For this review, take the finished solid that the model builds, in its own axes (mm). Face numbers are marked on the shaded views. A direction names the side the tool comes from. Coordinates: 2 decimals unless noted, no trailing zeros. Order: outer loops, then holes, each group sorted by start corner. A loop starts at its lowest first (then second) coordinate and runs counter-clockwise, first axis right, second up. Notation, with made-up numbers: (15.5, 48) -> (46.5, 48) arc R25 cw to (46.5, 79) -> close; hole circle Ø9 at (67.5, 81.5). An arc over 180 degrees is marked (long way). Return JSON: item names as keys, results as strings. Group by question number.
Item 1: Take a section at C-C (y = -26). Write out the cut boundary in (x, z).
Item 2: For line 1 along Y through (x, z) = (-312, 6); line 2 along X through (y, z) = (-67, 11); line 3 along Z through (x, y) = (312, -68), list the stretches that pass through material, from the lowest coordinate up.
Item 3: Take a section at B-B (x = 178.5). Write out the cut boundary in (y, z), then the cut area to 3 significant figures.
Item 4: Draft analysis for pull direction Z (two halves, no side actions). For the marked faces 1 and 2, state which applies: +Z half, -Z half, draft (parallel to the pull), parting line (faces both ways), or undercut.
Item 5: Take a section at D-D (z = 59.5). Write out the cut boundary in (x, y).
Item 6: Machinability: for the marked faces 3 and 4, which of the approach directions +Z, -Z, +X, -X, +Y, -Y give a long, thin tool a straight path to every point of the face, cutting with its end or side? Answer none if there is none.
Item 7: Take a section at A-A (y = -51). Write out the cut boundary in (x, z).
Item 8: Insertion check: pin 1 (4 mm diameter, centred on x = -326, z = 4, fed in from +Y); pin 2 (4 mm diameter, centred on x = 2, z = 13, fed in from -Y); pin 3 (0.8 mm diameter, centred on x = 312, y = -76.5, fed in from +Z). Each pin has a flat end and moves straight along its axis. Give the tip position at first contact, or say it passes through.
```python
from build123d import *

# Parameters (mm, degrees)
BASE_FLANGE1_DEPTH             = 102
EDGE_FLANGE1_STRIP_W           = 6
EDGE_FLANGE1_STRIP_H           = 1
EDGE_FLANGE1_STRIP_CUT_DEPTH   = 621.4
EDGE_FLANGE1_RELIEF_W          = 6.5
EDGE_FLANGE1_RELIEF_H          = 0.5
EDGE_FLANGE1_RELIEF_CUT_DEPTH  = 1
EDGE_FLANGE1_DEPTH             = 621.4
EDGE_FLANGE2_STRIP_W           = 6
EDGE_FLANGE2_STRIP_H           = 1
EDGE_FLANGE2_STRIP_CUT_DEPTH   = 621.4
EDGE_FLANGE2_DEPTH             = 621.4
EDGE_FLANGE3_STRIP_W           = 6
EDGE_FLANGE3_STRIP_H           = 1
EDGE_FLANGE3_STRIP_CUT_DEPTH   = 80
EDGE_FLANGE3_RELIEF_W          = 6.5
EDGE_FLANGE3_RELIEF_H          = 0.5
EDGE_FLANGE3_RELIEF_CUT_DEPTH  = 1
EDGE_FLANGE3_DEPTH             = 80
EDGE_FLANGE4_STRIP_W           = 6
EDGE_FLANGE4_STRIP_H           = 1
EDGE_FLANGE4_STRIP_CUT_DEPTH   = 80
EDGE_FLANGE4_DEPTH             = 80
EDGE_FLANGE5_STRIP_W           = 6
EDGE_FLANGE5_STRIP_H           = 1
EDGE_FLANGE5_STRIP_CUT_DEPTH   = 577.4
EDGE_FLANGE5_RELIEF_W          = 6.5
EDGE_FLANGE5_RELIEF_H          = 0.5
EDGE_FLANGE5_RELIEF_CUT_DEPTH  = 1
EDGE_FLANGE5_DEPTH             = 577.4
SKETCH25_R                     = 2.5
CUT_EXTRUDE1_DEPTH             = 3
SKETCH26_R                     = 2.5
CUT_EXTRUDE2_DEPTH             = 3
CUT_EXTRUDE2_DIRECTION_2_REACH = 661.221
EDGE_FLANGE7_STRIP_W           = 6
EDGE_FLANGE7_STRIP_H           = 1
EDGE_FLANGE7_STRIP_CUT_DEPTH   = 577.4
EDGE_FLANGE7_DEPTH             = 577.4
EDGE_FLANGE7_FLAT_DEPTH        = 1
SKETCH30_W                     = 21
SKETCH30_H                     = 65.6
CUT_EXTRUDE3_DEPTH             = 10
FILLET1_R                      = 2


# Sheet-metal steps are written as plain solids
with BuildPart() as part:
    # Sketch1 → Base-Flange1 (new body)
    with BuildSketch(Plane.XY):
        with BuildLine():
            Line((-330.7, -100), (-330.7, -15))
            ThreePointArc((-330.7, -15), (-326.306601718, -4.393398282), (-315.7, 0))
            Line((-315.7, 0), (315.7, 0))
            ThreePointArc((315.7, 0), (326.306601718, -4.393398282), (330.7, -15))
            Line((330.7, -15), (330.7, -100))
            Line((330.7, -100), (331.7, -100))
            Line((331.7, -100), (331.7, -15))
            ThreePointArc((331.7, -15), (327.013708499, -3.686291501), (315.7, 1))
            Line((315.7, 1), (-315.7, 1))
            ThreePointArc((-315.7, 1), (-327.013708499, -3.686291501), (-331.7, -15))
            Line((-331.7, -15), (-331.7, -100))
            Line((-331.7, -100), (-330.7, -100))
        make_face()
    extrude(amount=BASE_FLANGE1_DEPTH)

    # Edge-Flange1 strip (across the edge) → Edge-Flange1 strip cut (cut)
    with BuildSketch(Plane(origin=(-310.7, 0, 0), x_dir=(0, 0, 1), z_dir=(1, 0, 0))):
        with Locations((-2, -0.5)):
            Rectangle(EDGE_FLANGE1_STRIP_W, EDGE_FLANGE1_STRIP_H)
    extrude(amount=EDGE_FLANGE1_STRIP_CUT_DEPTH, mode=Mode.SUBTRACT)

    # Edge-Flange1 relief (on the sheet) → Edge-Flange1 relief cut (cut)
    with BuildSketch(Plane(origin=(-310.7, 0, 1), x_dir=(0, 0, 1), z_dir=(0, -1, 0))):
        with Locations((-2.75, 0.25)):
            Rectangle(EDGE_FLANGE1_RELIEF_W, EDGE_FLANGE1_RELIEF_H)
        with Locations((-2.75, -621.65)):
            Rectangle(EDGE_FLANGE1_RELIEF_W, EDGE_FLANGE1_RELIEF_H)
    extrude(amount=-EDGE_FLANGE1_RELIEF_CUT_DEPTH, mode=Mode.SUBTRACT)

    # Edge-Flange1 section (across the edge) → Edge-Flange1 (add)
    with BuildSketch(Plane(origin=(-310.7, 0, 0), x_dir=(0, 0, 1), z_dir=(1, 0, 0))):
        with BuildLine():
            Line((-1, 1), (-1, 19))
            Line((-1, 19), (0, 19))
            Line((0, 19), (0, 1))
            ThreePointArc((0, 1), (0.292893219, 0.292893219), (1, 0))
            Line((1, 0), (1, -1))
            ThreePointArc((1, -1), (-0.414213562, -0.414213562), (-1, 1))
        make_face()
    extrude(amount=EDGE_FLANGE1_DEPTH)

    # Edge-Flange2 strip (across the edge) → Edge-Flange2 strip cut (cut)
    with BuildSketch(Plane(origin=(-310.7, -19, 0), x_dir=(0, 1, 0), z_dir=(1, 0, 0))):
        with Locations((-1, -0.5)):
            Rectangle(EDGE_FLANGE2_STRIP_W, EDGE_FLANGE2_STRIP_H)
    extrude(amount=EDGE_FLANGE2_STRIP_CUT_DEPTH, mode=Mode.SUBTRACT)

    # Edge-Flange2 section (across the edge) → Edge-Flange2 (add)
    with BuildSketch(Plane(origin=(-310.7, -19, 0), x_dir=(0, 1, 0), z_dir=(1, 0, 0))):
        with BuildLine():
            Line((0, 1), (0, 12))
            Line((0, 12), (1, 12))
            Line((1, 12), (1, 1))
            ThreePointArc((1, 1), (1.292893219, 0.292893219), (2, 0))
            Line((2, 0), (2, -1))
            ThreePointArc((2, -1), (0.585786438, -0.414213562), (0, 1))
        make_face()
    extrude(amount=EDGE_FLANGE2_DEPTH)

    # Edge-Flange3 strip (across the edge) → Edge-Flange3 strip cut (cut)
    with BuildSketch(Plane(origin=(-330.7, -100, 0), x_dir=(0, 0, 1), z_dir=(0, 1, 0))):
        with Locations((-2, -0.5)):
            Rectangle(EDGE_FLANGE3_STRIP_W, EDGE_FLANGE3_STRIP_H)
    edge_flange3_strip_cut = extrude(amount=EDGE_FLANGE3_STRIP_CUT_DEPTH, mode=Mode.SUBTRACT)

    # Edge-Flange3 relief (on the sheet) → Edge-Flange3 relief cut (cut)
    with BuildSketch(Plane(origin=(-330.7, -100, 1), x_dir=(0, 0, 1), z_dir=(1, 0, 0))):
        with Locations((-2.75, -80.25)):
            Rectangle(EDGE_FLANGE3_RELIEF_W, EDGE_FLANGE3_RELIEF_H)
    edge_flange3_relief_cut = extrude(amount=-EDGE_FLANGE3_RELIEF_CUT_DEPTH, mode=Mode.SUBTRACT)

    # Edge-Flange3 section (across the edge) → Edge-Flange3 (add)
    with BuildSketch(Plane(origin=(-330.7, -100, 0), x_dir=(0, 0, 1), z_dir=(0, 1, 0))):
        with BuildLine():
            Line((-1, 1), (-1, 19))
            Line((-1, 19), (0, 19))
            Line((0, 19), (0, 1))
            ThreePointArc((0, 1), (0.292893219, 0.292893219), (1, 0))
            Line((1, 0), (1, -1))
            ThreePointArc((1, -1), (-0.414213562, -0.414213562), (-1, 1))
        make_face()
    edge_flange3 = extrude(amount=EDGE_FLANGE3_DEPTH)

    # Edge-Flange4 strip (across the edge) → Edge-Flange4 strip cut (cut)
    with BuildSketch(Plane(origin=(-311.7, -100, 0), x_dir=(-1, 0, 0), z_dir=(0, 1, 0))):
        with Locations((-1, -0.5)):
            Rectangle(EDGE_FLANGE4_STRIP_W, EDGE_FLANGE4_STRIP_H)
    edge_flange4_strip_cut = extrude(amount=EDGE_FLANGE4_STRIP_CUT_DEPTH, mode=Mode.SUBTRACT)

    # Edge-Flange4 section (across the edge) → Edge-Flange4 (add)
    with BuildSketch(Plane(origin=(-311.7, -100, 0), x_dir=(-1, 0, 0), z_dir=(0, 1, 0))):
        with BuildLine():
            Line((0, 1), (0, 12))
            Line((0, 12), (1, 12))
            Line((1, 12), (1, 1))
            ThreePointArc((1, 1), (1.292893219, 0.292893219), (2, 0))
            Line((2, 0), (2, -1))
            ThreePointArc((2, -1), (0.585786438, -0.414213562), (0, 1))
        make_face()
    edge_flange4 = extrude(amount=EDGE_FLANGE4_DEPTH)

    # Mirror1: Edge-Flange3 strip cut, Edge-Flange3 relief cut, Edge-Flange3, Edge-Flange4 strip cut, Edge-Flange4 across plane
    add(edge_flange3_strip_cut.mirror(Plane(origin=(0, 0, 0), x_dir=(0, 0, 1), z_dir=(1, 0, 0))), mode=Mode.SUBTRACT)
    add(edge_flange3_relief_cut.mirror(Plane(origin=(0, 0, 0), x_dir=(0, 0, 1), z_dir=(1, 0, 0))), mode=Mode.SUBTRACT)
    add(edge_flange3.mirror(Plane(origin=(0, 0, 0), x_dir=(0, 0, 1), z_dir=(1, 0, 0))))
    add(edge_flange4_strip_cut.mirror(Plane(origin=(0, 0, 0), x_dir=(0, 0, 1), z_dir=(1, 0, 0))), mode=Mode.SUBTRACT)
    add(edge_flange4.mirror(Plane(origin=(0, 0, 0), x_dir=(0, 0, 1), z_dir=(1, 0, 0))))

    # Edge-Flange5 strip (across the edge) → Edge-Flange5 strip cut (cut)
    with BuildSketch(Plane(origin=(288.7, 0, 102), x_dir=(0, 0, -1), z_dir=(-1, 0, 0))):
        with Locations((-2, -0.5)):
            Rectangle(EDGE_FLANGE5_STRIP_W, EDGE_FLANGE5_STRIP_H)
    extrude(amount=EDGE_FLANGE5_STRIP_CUT_DEPTH, mode=Mode.SUBTRACT)

    # Edge-Flange5 relief (on the sheet) → Edge-Flange5 relief cut (cut)
    with BuildSketch(Plane(origin=(288.7, 0, 101), x_dir=(0, 0, -1), z_dir=(0, -1, 0))):
        with Locations((-2.75, 0.25)):
            Rectangle(EDGE_FLANGE5_RELIEF_W, EDGE_FLANGE5_RELIEF_H)
        with Locations((-2.75, -577.65)):
            Rectangle(EDGE_FLANGE5_RELIEF_W, EDGE_FLANGE5_RELIEF_H)
    extrude(amount=-EDGE_FLANGE5_RELIEF_CUT_DEPTH, mode=Mode.SUBTRACT)

    # Edge-Flange5 section (across the edge) → Edge-Flange5 (add)
    with BuildSketch(Plane(origin=(288.7, 0, 102), x_dir=(0, 0, -1), z_dir=(-1, 0, 0))):
        with BuildLine():
            Line((-1, 1), (-1, 35.5))
            Line((-1, 35.5), (0, 35.5))
            Line((0, 35.5), (0, 1))
            ThreePointArc((0, 1), (0.292893219, 0.292893219), (1, 0))
            Line((1, 0), (1, -1))
            ThreePointArc((1, -1), (-0.414213562, -0.414213562), (-1, 1))
        make_face()
    extrude(amount=EDGE_FLANGE5_DEPTH)

    # Sketch25 → Cut-Extrude1 (cut)
    with BuildSketch(Plane.XZ.offset(19)):
        with Locations(Location((-249.7, 6, 0), (0, 0, 270))):
            Circle(SKETCH25_R)
        with Locations(Location((-69.7, 6, 0), (0, 0, 270))):
            Circle(SKETCH25_R)
        with Locations(Location((110.3, 6, 0), (0, 0, 270))):
            Circle(SKETCH25_R)
        with Locations(Location((290.3, 6, 0), (0, 0, 270))):
            Circle(SKETCH25_R)
        with Locations((470.3, 6)):
            Circle(SKETCH25_R)
        with Locations((650.3, 6)):
            Circle(SKETCH25_R)
        with Locations((830.3, 6)):
            Circle(SKETCH25_R)
    extrude(amount=-CUT_EXTRUDE1_DEPTH, mode=Mode.SUBTRACT)

    # Sketch26 → Cut-Extrude2 (cut)
    with BuildSketch(Plane(origin=(-311.7, 0, 0), x_dir=(0, 0, -1), z_dir=(1, 0, 0))):
        with Locations((-6, -68)):
            Circle(SKETCH26_R)
    extrude(amount=-CUT_EXTRUDE2_DEPTH, mode=Mode.SUBTRACT)

    # Cut-Extrude2 direction 2: up to this face of the body (flat: up to its plane)
    cut_extrude2_direction_2_end = Plane(part.part.faces().sort_by_distance((312.7, -60, 6.5))[0])
    # Sketch26 → Cut-Extrude2 direction 2 (cut, up to the picked face)
    with BuildSketch(Plane(origin=(-311.7, 0, 0), x_dir=(0, 0, -1), z_dir=(1, 0, 0)), mode=Mode.PRIVATE) as cut_extrude2_direction_2_sk1:
        with Locations((-6, -68)):
            Circle(SKETCH26_R)
    cut_extrude2_direction_2_tool1 = split(extrude(cut_extrude2_direction_2_sk1.sketch, amount=CUT_EXTRUDE2_DIRECTION_2_REACH, mode=Mode.PRIVATE), bisect_by=cut_extrude2_direction_2_end, keep=Keep.BOTH, mode=Mode.PRIVATE)
    add(cut_extrude2_direction_2_tool1.solids().sort_by(Axis((-311.7, -68, 6), (1, 0, 0)))[0], mode=Mode.SUBTRACT)

    # Edge-Flange7 strip (across the edge) → Edge-Flange7 strip cut (cut)
    with BuildSketch(Plane(origin=(288.7, -35.5, 102), x_dir=(0, 1, 0), z_dir=(-1, 0, 0))):
        with Locations((-1, -0.5)):
            Rectangle(EDGE_FLANGE7_STRIP_W, EDGE_FLANGE7_STRIP_H)
    extrude(amount=EDGE_FLANGE7_STRIP_CUT_DEPTH, mode=Mode.SUBTRACT)

    # Edge-Flange7 bend section (across the edge) → Edge-Flange7 (add)
    with BuildSketch(Plane(origin=(288.7, -35.5, 102), x_dir=(0, 1, 0), z_dir=(-1, 0, 0))):
        with BuildLine():
            Line((0, 1), (1, 1))
            ThreePointArc((1, 1), (1.292893219, 0.292893219), (2, 0))
            Line((2, 0), (2, -1))
            ThreePointArc((2, -1), (0.585786438, -0.414213562), (0, 1))
        make_face()
    extrude(amount=EDGE_FLANGE7_DEPTH)

    # Edge-Flange7 profile (on flange) → Edge-Flange7 flat (add)
    with BuildSketch(Plane(origin=(0, -35.5, 102), x_dir=(1, 0, 0), z_dir=(0, 1, 0))):
        with BuildLine():
            Line((-288.7, 1), (288.7, 1))
            Line((288.7, 1), (288.7, 28))
            ThreePointArc((288.7, 28), (287.821320344, 30.121320344), (285.7, 31))
            Line((285.7, 31), (-285.7, 31))
            ThreePointArc((-285.7, 31), (-287.821320344, 30.121320344), (-288.7, 28))
            Line((-288.7, 28), (-288.7, 1))
        make_face()
    extrude(amount=EDGE_FLANGE7_FLAT_DEPTH)

    # Sketch30 → Cut-Extrude3 (cut)
    with BuildSketch(Plane(origin=(331.7, 0, 0), x_dir=(0, 0, -1), z_dir=(1, 0, 0))):
        with Locations((-91.5, -67.2)):
            Rectangle(SKETCH30_W, SKETCH30_H)
    extrude(amount=-CUT_EXTRUDE3_DEPTH, mode=Mode.SUBTRACT)

    # Fillet1
    fillet1_edges = [part.edges().sort_by_distance(p)[0] for p in [
        (331.2, -34.4, 102),
    ]]
    fillet(fillet1_edges, radius=FILLET1_R)


solid = part.part
```
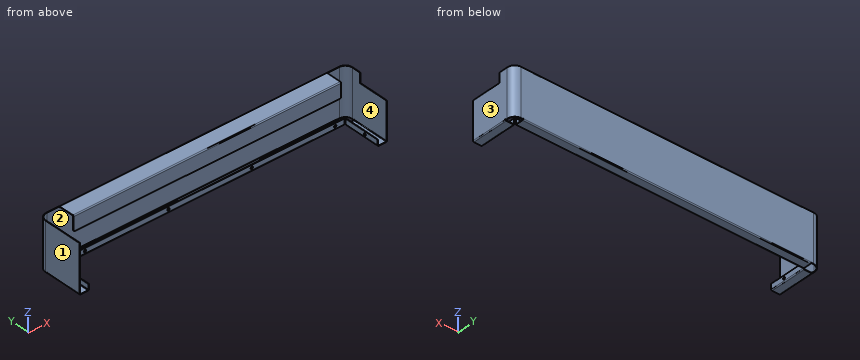
Findings below:
{
 "1": {"outline": "(-331.7, 1) arc R2 ccw to (-329.7, -1) -> (-313.7, -1) arc R2 ccw to (-311.7, 1) -> (-311.7, 12) -> (-312.7, 12) -> (-312.7, 1) arc R1 cw to (-313.7, 0) -> (-329.7, 0) arc R1 cw to (-330.7, 1) -> (-330.7, 102) -> (-331.7, 102) -> close; (-288.7, 102) -> (288.7, 102) -> (288.7, 103) -> (-288.7, 103) -> close; (311.7, 1) arc R2 ccw to (313.7, -1) -> (329.7, -1) arc R2 ccw to (331.7, 1) -> (331.7, 102) -> (330.7, 102) -> (330.7, 1) arc R1 cw to (329.7, 0) -> (313.7, 0) arc R1 cw to (312.7, 1) -> (312.7, 12) -> (311.7, 12) -> close"},
 "2": {"line 1": "y = -100 to -70.5, -65.5 to -20, 0 to 1", "line 2": "x = -331.7 to -330.7, -312.7 to -311.7, 311.7 to 312.7, 330.7 to 331.7", "line 3": "z = -0.05 to 3.5, 8.5 to 12"},
 "3": {"outline": "(-35.5, 71) -> (-34.5, 71) -> (-34.5, 101) arc R1 cw to (-33.5, 102) -> (-1, 102) arc R1 cw to (0, 101) -> (0, 1) arc R1 cw to (-1, 0) -> (-17, 0) arc R1 cw to (-18, 1) -> (-18, 12) -> (-19, 12) -> (-19, 1) arc R2 ccw to (-17, -1) -> (-1, -1) arc R2 ccw to (1, 1) -> (1, 101) arc R2 ccw to (-1, 103) -> (-33.5, 103) arc R2 ccw to (-35.5, 101) -> close", "area": "199 mm2"},
 "4": {"face 1": "draft", "face 2": "undercut"},
 "5": {"outline": "(-331.7, -100) -> (-330.7, -100) -> (-330.7, -15) arc R15 cw to (-315.7, 0) -> (315.7, 0) arc R15 cw to (330.7, -15) -> (330.7, -100) -> (331.7, -100) -> (331.7, -15) arc R16 ccw to (315.7, 1) -> (-315.7, 1) arc R16 ccw to (-331.7, -15) -> close"},
 "6": {"face 3": "+Z, -Z, +X, +Y, -Y", "face 4": "+Z, -Y"},
 "7": {"outline": "(-331.7, 1) arc R2 ccw to (-329.7, -1) -> (-313.7, -1) arc R2 ccw to (-311.7, 1) -> (-311.7, 12) -> (-312.7, 12) -> (-312.7, 1) arc R1 cw to (-313.7, 0) -> (-329.7, 0) arc R1 cw to (-330.7, 1) -> (-330.7, 102) -> (-331.7, 102) -> close; (311.7, 1) arc R2 ccw to (313.7, -1) -> (329.7, -1) arc R2 ccw to (331.7, 1) -> (331.7, 81) -> (330.7, 81) -> (330.7, 1) arc R1 cw to (329.7, 0) -> (313.7, 0) arc R1 cw to (312.7, 1) -> (312.7, 12) -> (311.7, 12) -> close"},
 "8": {"pin 1": "stops at y = -1.32", "pin 2": "stops at y = -19", "pin 3": "stops at z = 12"}
}
